from build123d import *
from OCP.BRepFilletAPI import BRepFilletAPI_MakeChamfer

# Parameters (mm, degrees)
SKETCH_1_R      = 16
SKETCH_1_R_2    = 10
EXTRUDE_1_DEPTH = 7
SKETCH_1_3_R    = 17.5
SKETCH_1_3_R_2  = 16
EXTRUDE_2_DEPTH = 1.5
CHAMFER_1_SIZE  = 0.2
CHAMFER_1_SIZE2 = 0.115470054


with BuildPart() as part:
    # Sketch 1 → Extrude 1 (new body)
    with BuildSketch(Plane(origin=(0, 0, 0), x_dir=(1, 0, 0), z_dir=(0, 1, 0))):
        with Locations(Location((0, 0, 0), (0, 0, 270))):
            Circle(SKETCH_1_R)
        with Locations(Location((0, 0, 0), (0, 0, 270))):
            Circle(SKETCH_1_R_2, mode=Mode.SUBTRACT)
    extrude(amount=EXTRUDE_1_DEPTH)

    # Sketch 1_3 → Extrude 2 (add)
    with BuildSketch(Plane(origin=(0, 0, 0), x_dir=(1, 0, 0), z_dir=(0, 1, 0))):
        with Locations(Location((0, 0, 0), (0, 0, 270))):
            Circle(SKETCH_1_3_R)
        with Locations(Location((0, 0, 0), (0, 0, 270))):
            Circle(SKETCH_1_3_R_2, mode=Mode.SUBTRACT)
    extrude(amount=EXTRUDE_2_DEPTH)

    # Chamfer 1: one chamfer whose edges measure the first distance from different faces: ONE call of the kernel's chamfer builder (chamfer() names one face for all edges)
    chamfer_1_edges_1 = [part.edges().sort_by_distance(p)[0] for p in [
        (0, 7, -16),
    ]]
    chamfer_1_side_1 = [part.faces().sort_by_distance(p)[0] for p in [
        (0, 4.25, -16),
    ]]
    chamfer_1_edges_2 = [part.edges().sort_by_distance(p)[0] for p in [
        (0, 0, -17.5),
    ]]
    chamfer_1_side_2 = [part.faces().sort_by_distance(p)[0] for p in [
        (0, 0, -17.005025253),
    ]]
    chamfer_1 = BRepFilletAPI_MakeChamfer(part.part.solid().wrapped)
    for e in chamfer_1_edges_1:
        chamfer_1.Add(CHAMFER_1_SIZE, CHAMFER_1_SIZE2, e.wrapped, chamfer_1_side_1[0].wrapped)  # the first distance lies on this face
    for e in chamfer_1_edges_2:
        chamfer_1.Add(CHAMFER_1_SIZE, CHAMFER_1_SIZE2, e.wrapped, chamfer_1_side_2[0].wrapped)  # the first distance lies on this face
    add(Compound.cast(chamfer_1.Shape()), mode=Mode.REPLACE)


solid = part.part
Check sheet for the modelled part. Datum: model origin and axes. Units: mm. Round coordinates to 2 decimals unless told otherwise and drop trailing zeros. Order: outer loops, then holes, each group sorted by start corner. A loop starts at its lowest first (then second) coordinate and runs counter-clockwise, first axis right, second up.
(1) Draft check along X on faces 1 (the flat face through (-14.2, 1.5, 7.7)), 2 (the cylindrical face through (-15.62, 4.11, -3.47)), 3 (the cylindrical face through (-9.76, 3.45, -2.17)). Enter one of: pulls with the +X half, pulls with the -X half, needs draft (parallel to the pull), parting line crosses it, or undercut.
(2) Go/stop test with flat-tipped pins: P1, Ø2, axis at x = -4, y = 6, coming from the +Z side; P2, Ø1.5, axis at x = -14, y = 5, coming from the +Z side; P3, Ø2, axis at x = 5.5, y = 2, coming from the -Z side. Record where each tip stops, or that it passes through.
(3) Cross-section at B-B, the plane z = 0. Enter the section's corners in (x, y), and give its area (3 significant figures).
(4) Cross-section at A-A, the plane x = 0. Enter the section's corners in (y, z), and give its area (3 significant figures).
(5) Scan lines: probe 1 along X at (y, z) = (3.5, 0); probe 2 along X at (y, z) = (5.5, -6.5); probe 3 along Z at (x, y) = (-7.5, 1.25). Record each from-to range of solid material in increasing order.
(6) Cross-section at C-C, the plane y = 4. Enter the section's corners in (x, z), and give its area (3 significant figures).
Check sheet entries:
1. face 1: needs draft
1. face 2: parting line crosses it
1. face 3: undercut
2. P1: stops at z = 15.72
2. P2: stops at z = 8.97
2. P3: stops at z = -16.88
3. outline: (-17.5, 0.12) - (-17.3, 0) - (-10, 0) - (-10, 7) - (-15.88, 7) - (-16, 6.8) - (-16, 1.5) - (-17.5, 1.5) - close; (10, 0) - (17.3, 0) - (17.5, 0.12) - (17.5, 1.5) - (16, 1.5) - (16, 6.8) - (15.88, 7) - (10, 7) - close
3. area: 88.5 mm2
4. outline: (0, -17.3) - (0.12, -17.5) - (1.5, -17.5) - (1.5, -16) - (6.8, -16) - (7, -15.88) - (7, -10) - (0, -10) - close; (0, 10) - (7, 10) - (7, 15.88) - (6.8, 16) - (1.5, 16) - (1.5, 17.5) - (0.12, 17.5) - (0, 17.3) - close
4. area: 88.5 mm2
5. probe 1: x = -16 to -10, 10 to 16
5. probe 2: x = -14.62 to -7.6, 7.6 to 14.62
5. probe 3: z = -15.81 to -6.61, 6.61 to 15.81
6. outline: circle Ø32 at (0, 0); hole circle Ø20 at (0, 0)
6. area: 490 mm2
